CAD build for the part. Positions are in the model's coordinates, mm. A direction names the side the tool comes from. Round coordinates to 2 decimals unless told otherwise and drop trailing zeros. Write each loop counter-clockwise with the first axis right and the second up, starting at its lowest first coordinate (ties: lowest second). Pieces come first, ordered by that corner, then holes. Notation, with made-up numbers: (-5.5, 26.5) -> (-0.5, 26.5) arc R20 cw to (-0.5, 34.5) -> close; hole circle Ø8 at (17, 23). An arc over 180 degrees is marked (long way). Put each result on its own line as item: value. Start each with the question number.
1. 3-axis set-ups, long thin cutter, end or side, ignore diameter. For faces 1 (the cylindrical face through (-5.786, 5.305, 3.756)), 2 (the cylindrical face through (4.626, 1.457, 0.046)): which of +Z, -Z, +X, -X, +Y, -Y reach the whole face in a straight line?
2. Flat gauge pins, fed straight in: P1, Ø4, axis at y = 5, z = 2.5, coming from the +X side; P2, Ø3, axis at x = -0.5, z = -2.5, coming from the +Y side; P3, Ø1.5, axis at y = 0.5, z = -2, coming from the -X side. Where does each tip first touch, or does it go through?
3. Saw through at C-C on z = 0. List the corners of the cut face in (x, y).
4. Saw through at A-A on y = 0. List the corners of the cut face in (x, z), and give its area (3 significant figures).
5. Saw through at D-D on y = 6.5. List the corners of the cut face in (x, z), and give its area (3 significant figures).
6. Pull direction Y, two halves, no side cores. Call faces 3 (the flat face through (0, -2, -4.2)), 4 (the cylindrical face through (-5.786, 5.305, -3.756)), 5 (the cylindrical face through (0.715, -1.375, -0.059)): pulls with the +Y half, pulls with the -Y half, needs draft (parallel to the pull), parting line crosses it, or undercut.
7. Drill centre lines: line 1 (Z direction, x = 3.25, y = 6.75); line 2 (Y direction, x = 0, z = -1); line 3 (X direction, y = 3.5, z = 1.25). Where is each one in solid material? Low to high. Write a range as from..to.
from build123d import *

# Parameters (mm, degrees)
SKETCH1_R           = 4.85
SKETCH1_R_2         = 1.55
BOSS_EXTRUDE1_DEPTH = 4.2
BOSS_EXTRUDE2_START = 4.2
SKETCH1_3_R         = 7.85
SKETCH1_3_R_2       = 4.85
BOSS_EXTRUDE2_DEPTH = 0.9
BOSS_EXTRUDE3_START = -4.2
SKETCH1_4_R         = 7.85
SKETCH1_4_R_2       = 4.85
BOSS_EXTRUDE3_DEPTH = 0.9


with BuildPart() as part:
    # Sketch1 → Boss-Extrude1 (new body, symmetric)
    with BuildSketch(Plane.XY):
        Circle(SKETCH1_R)
        Circle(SKETCH1_R_2, mode=Mode.SUBTRACT)
    extrude(amount=BOSS_EXTRUDE1_DEPTH, both=True)

    # Sketch1<3> → Boss-Extrude2 (add)
    with BuildSketch(Plane.XY.offset(BOSS_EXTRUDE2_START)):
        Circle(SKETCH1_3_R)
        Circle(SKETCH1_3_R_2, mode=Mode.SUBTRACT)
    extrude(amount=-BOSS_EXTRUDE2_DEPTH)

    # Sketch1<4> → Boss-Extrude3 (add)
    with BuildSketch(Plane.XY.offset(BOSS_EXTRUDE3_START)):
        Circle(SKETCH1_4_R)
        Circle(SKETCH1_4_R_2, mode=Mode.SUBTRACT)
    extrude(amount=BOSS_EXTRUDE3_DEPTH)


solid = part.part
Return value:
1. face 1: +Z, -Z
1. face 2: none
2. P1: stops at x = 7.18
2. P2: stops at y = 7.85
2. P3: stops at x = -4.85
3. outline: circle Ø9.7 at (0, 0); hole circle Ø3.1 at (0, 0)
4. outline: (-7.85, -4.2) -> (-1.55, -4.2) -> (-1.55, 4.2) -> (-7.85, 4.2) -> (-7.85, 3.3) -> (-4.85, 3.3) -> (-4.85, -3.3) -> (-7.85, -3.3) -> close; (1.55, -4.2) -> (7.85, -4.2) -> (7.85, -3.3) -> (4.85, -3.3) -> (4.85, 3.3) -> (7.85, 3.3) -> (7.85, 4.2) -> (1.55, 4.2) -> close
4. area: 66.2 mm^2
5. outline: (-4.4, -4.2) -> (4.4, -4.2) -> (4.4, -3.3) -> (-4.4, -3.3) -> close; (-4.4, 3.3) -> (4.4, 3.3) -> (4.4, 4.2) -> (-4.4, 4.2) -> close
5. area: 15.8 mm^2
6. face 3: needs draft
6. face 4: parting line crosses it
6. face 5: undercut
7. line 1: z = -4.2..-3.3, 3.3..4.2
7. line 2: y = -4.85..-1.55, 1.55..4.85
7. line 3: x = -3.36..3.36
